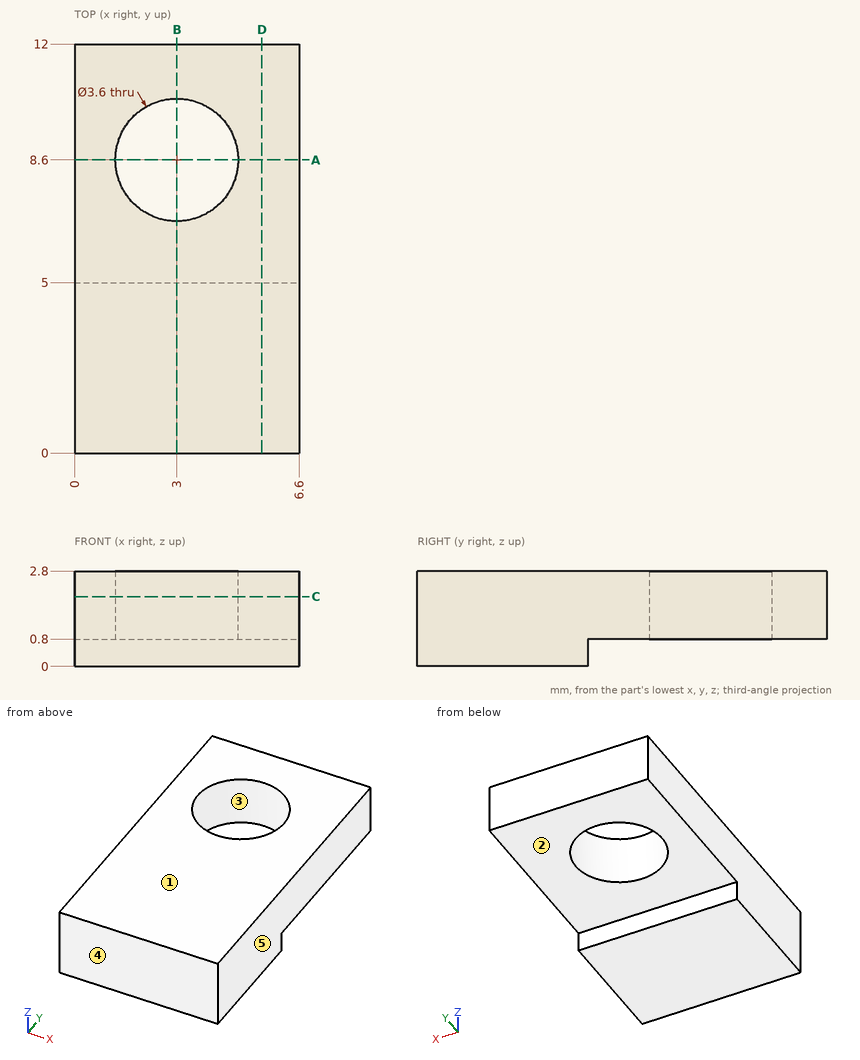
Geometry: see drawing. Coordinates: mm, zero at the bounding-box minimum. A direction names the side the tool comes from. Coordinates: 2 decimals unless noted, no trailing zeros. Order: outer loops, then holes, each group sorted by start corner. A loop starts at its lowest first (then second) coordinate and runs counter-clockwise, first axis right, second up. Notation, with made-up numbers: (-26, -25) - (28, -25) arc R20 ccw to (28, 13) - close; hole circle Ø10 at (43, 66). An arc over 180 degrees is marked (long way). Use one line per item in the form item = value.
1) Ray query, L1, parallel to Y at x = 3, z = 2.2; L2, parallel to X at y = 8.6, z = 1.7; L3, parallel to Z at x = 2.25, y = 6.25. Return the intervals inside material, ascending.
Solutions:
L1 = 0 to 6.8, 10.4 to 12
L2 = 0 to 1.2, 4.8 to 6.6
L3 = 0.8 to 2.8
2) Section D-D (x = 5.5). Return loops of the section in (y, z), then the cut area to 3 significant figures.
Solutions:
outline = (0, 0) - (5, 0) - (5, 0.8) - (12, 0.8) - (12, 2.8) - (0, 2.8) - close
area = 28.0 mm^2
3) Section A-A (y = 8.6). Return loops of the section in (x, z).
Solutions:
outline = (0, 0.8) - (1.2, 0.8) - (1.2, 2.8) - (0, 2.8) - close; (4.8, 0.8) - (6.6, 0.8) - (6.6, 2.8) - (4.8, 2.8) - close
4) Set-up query: the marked faces 1 and 2. Return all of +Z, -Z, +X, -X, +Y, -Y with unobstructed straight access to the full face (end or side cutting, diameter ignored); none if empty.
Solutions:
face_1 = +Z, +X, -X, +Y, -Y
face_2 = -Z, +X, -X, +Y
5) Section C-C (z = 2.05). Return loops of the section in (x, y).
Solutions:
outline = (0, 0) - (6.6, 0) - (6.6, 12) - (0, 12) - close; hole circle Ø3.6 at (3, 8.6)
6) Pin query (flat end, axial travel): pin 1 (1.5 mm diameter, centred on y = 9, z = 0.5, fed in from +X); pin 2 (1 mm diameter, centred on x = 3.5, y = 9.5, fed in from +Z); pin 3 (2 mm diameter, centred on x = 4.5, y = 8.5, fed in from -Z). Return the tip coordinate at first contact, or that it passes through.
Solutions:
pin_1 = 6.6
pin_2 = through
pin_3 = 0.8
7) Mould query, pull axis X, two halves, no side actions, for the marked faces 3, 4 and 5. Classes: +X half, -X half, draft (parallel to the pull), parting line (faces both ways), or undercut.
Solutions:
face_3 = undercut
face_4 = draft
face_5 = +X half
8) Section B-B (x = 3). Return loops of the section in (y, z), then the cut area to 3 significant figures.
Solutions:
outline = (0, 0) - (5, 0) - (5, 0.8) - (6.8, 0.8) - (6.8, 2.8) - (0, 2.8) - close; (10.4, 0.8) - (12, 0.8) - (12, 2.8) - (10.4, 2.8) - close
area = 20.8 mm^2
